Could you check a few things on this drawing? It's one solid part, dimensions in mm from its lowest x, y, z. A direction names the side the tool comes from. Round coordinates to 2 decimals unless told otherwise and drop trailing zeros. Write each loop counter-clockwise with the first axis right and the second up, starting at its lowest first coordinate (ties: lowest second). Pieces come first, ordered by that corner, then holes. Notation, with made-up numbers: (62.25, 54) -> (95.25, 54) arc R3 cw to (95.25, 58) -> close; hole circle Ø11 at (-7, -24.5). An arc over 180 degrees is marked (long way). Put each result on its own line as item: value. Start each with the question number.
1) I want a section at B-B, the plane x = 4.5. List the corners of the cut face in (y, z) for me.
2) If I drill on line 1 along X through (y, z) = (1.25, 10); line 2 along Z through (x, y) = (8.25, 8.25); line 3 along Y through (x, z) = (2.75, 11.5), over which ranges is the centre line in solid material (lowest first)? Write a range as [from, to].
3) I want a section at C-C, the plane z = 8. List the corners of the cut face in (x, y) for me.
4) We'd pull the mould along Z, two halves only. Please class the marked faces 3, 4 and 5: released by +Z, released by -Z, zero draft, split by the parting line, or undercut.
5) Will this pin go through, and if not, where does the flat tip stop? P1, Ø3, axis at x = 8.5, z = 11, coming from the +Y side.
6) Which directions (+Z, -Z, +X, -X, +Y, -Y) give clear straight access to the entire face, cutting with the end or side of a thin tool? Please do the marked faces 1 and 2.
7) I want a section at A-A, the plane y = 5. List the corners of the cut face in (x, z) for me.
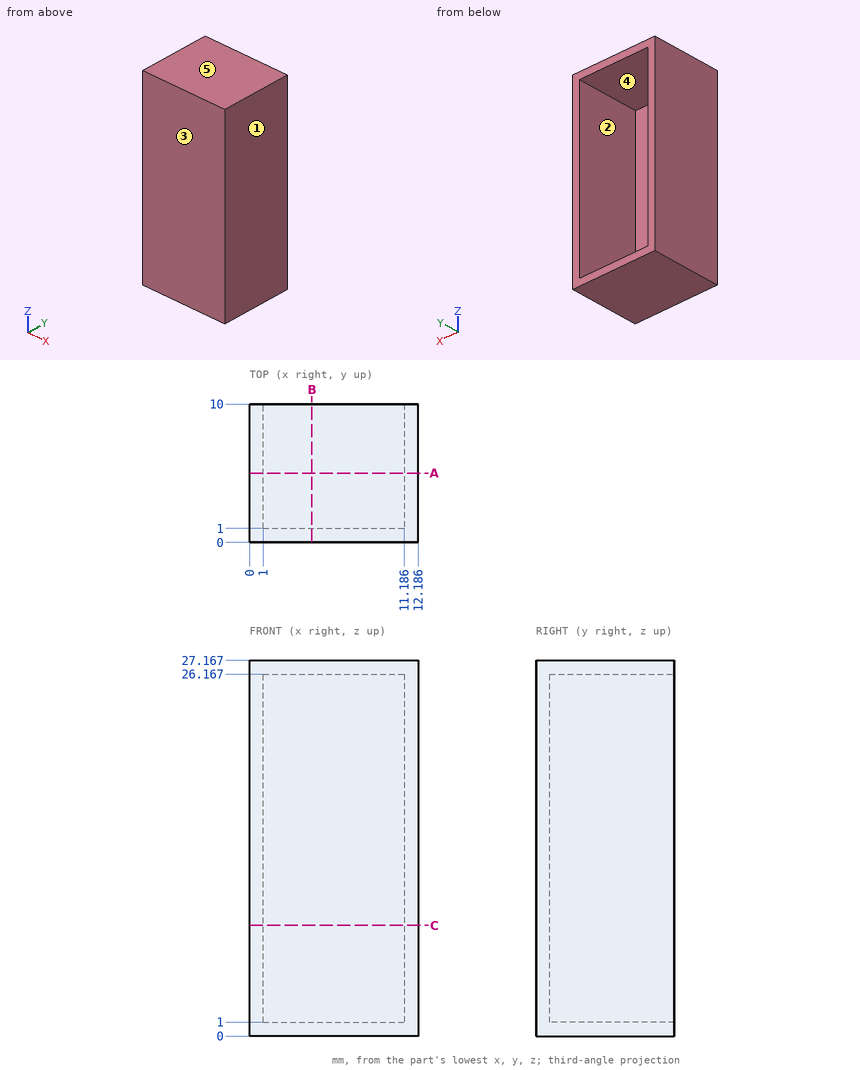
Findings:
1. outline: (0, 0) -> (10, 0) -> (10, 1) -> (1, 1) -> (1, 26.17) -> (10, 26.17) -> (10, 27.17) -> (0, 27.17) -> close
2. line 1: x = [0, 1], [11.19, 12.19]
2. line 2: z = [0, 1], [26.17, 27.17]
2. line 3: y = [0, 1]
3. outline: (0, 0) -> (12.19, 0) -> (12.19, 10) -> (11.19, 10) -> (11.19, 1) -> (1, 1) -> (1, 10) -> (0, 10) -> close
4. face 3: zero draft
4. face 4: undercut
4. face 5: released by +Z
5. P1: stops at y = 1
6. face 1: +Z, -Z, +X, +Y, -Y
6. face 2: +Y
7. outline: (0, 0) -> (12.19, 0) -> (12.19, 27.17) -> (0, 27.17) -> close; hole (1, 1) -> (11.19, 1) -> (11.19, 26.17) -> (1, 26.17) -> close
